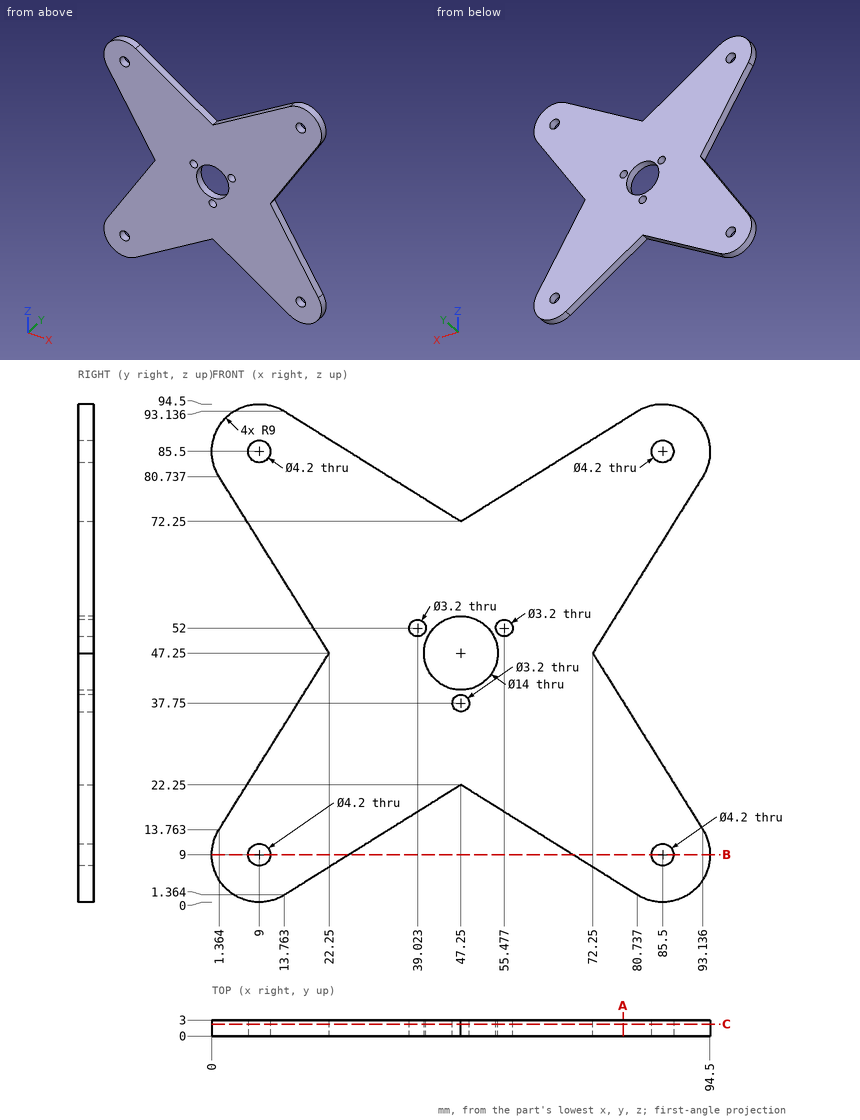
Could you check a few things on this drawing? It's one solid part, dimensions in mm from its lowest x, y, z. Coordinates: 2 decimals unless noted, no trailing zeros. Order: outer loops, then holes, each group sorted by start corner. A loop starts at its lowest first (then second) coordinate and runs counter-clockwise, first axis right, second up. Notation, with made-up numbers: M 44.5,4.5 L 69.5,4.5 A17 cw 69.5,25.5 Z; hole C -20.75,16 d6. An arc over 180 degrees is marked long. Answer as a JSON object with one key per item and string values. Group by question number.
(1) Suppose I cut it at A-A, the plane x = 78. Please give me the cut outline in (y, z).
(2) I need wall thicknesses on probe 1 along X at (y, z) = (2.4, 85.5) (1 decimal); probe 2 along X at (y, z) = (0.95, 85) (1 decimal); probe 3 along Z at (x, y) = (89, 1.85) (1 decimal). Which ranges of each line are inside material? Lowest first, please.
(3) For pin 1 (4 mm diameter, centred on x = 85.5, z = 9, fed in from +Y) (3 decimals); pin 2 (1 mm diameter, centred on x = 58, y = 2, fed in from -Z), each with a flat end and sliding along its axis, tell me the tip position at first contact or that it passes through.
(4) Suppose I cut it at B-B, the plane z = 9. Please give me the cut outline in (x, y).
(5) Suppose I cut it at C-C, the plane y = 2.25. State how many separate pieces and enclosed holes the cut face has, then the cut area to 3 significant figures.
Values found:
{
 "1": {"outline": "M 0,3.07 L 3,3.07 L 3,38.03 L 0,38.03 Z; M 0,56.47 L 3,56.47 L 3,91.43 L 0,91.43 Z"},
 "2": {"probe 1": "x = 0 to 6.9, 11.1 to 26, 68.5 to 83.4, 87.6 to 94.5", "probe 2": "x = 0 to 7, 11 to 26.8, 67.7 to 83.5, 87.5 to 94.5", "probe 3": "z = 0.7 to 20.4, 74.1 to 93.8"},
 "3": {"pin 1": "passes through", "pin 2": "stops at z = 15.23"},
 "4": {"outline": "M 0,0 L 6.9,0 L 6.9,3 L 0,3 Z; M 11.1,0 L 26.01,0 L 26.01,3 L 11.1,3 Z; M 68.49,0 L 83.4,0 L 83.4,3 L 68.49,3 Z; M 87.6,0 L 94.5,0 L 94.5,3 L 87.6,3 Z"},
 "5": {"separate pieces": "1", "enclosed holes": "8", "area": "5,450 mm^2"}
}
